Geometry check sheet. Reference: drawing and pictorial views, mm from the part's lowest x, y, z. Give positions to 0.01 mm unless a question says otherwise; leave off trailing zeros. Write each loop counter-clockwise with the first axis right and the second up, starting at its lowest first coordinate (ties: lowest second). Pieces come first, ordered by that corner, then holes. Notation, with made-up numbers: (20.5, -22) - (62.5, -22) arc R16 cw to (62.5, -5) - close; hole circle Ø8 at (41, 8.5). An arc over 180 degrees is marked (long way). Put each result on its own line as item: value.
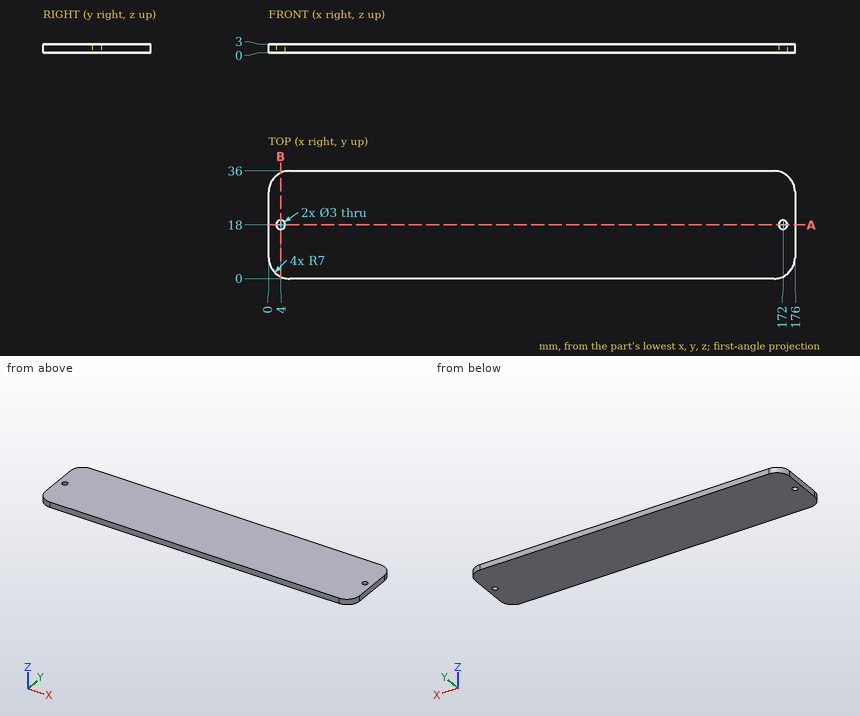
Q1. Go/stop test with a flat-tipped pin: pin 1 Ø1 at (y, z) = (5, 0.5) entering from +X. Record where the tip stops, or that it passes through.
Answers follow:
pin 1: stops at x = 175.84
Q2. Section check B-B, the plane x = 4. Record the cut outline in (y, z).
Answers follow:
outline: (0.68, 0) - (16.5, 0) - (16.5, 3) - (0.68, 3) - close; (19.5, 0) - (35.32, 0) - (35.32, 3) - (19.5, 3) - close
Q3. Scan lines: line 1 along Y through (x, z) = (4, 1.25); line 2 along X through (y, z) = (2, 2.6); line 3 along X through (y, z) = (33, 2.35). Record each from-to range of solid material in increasing order.
Answers follow:
line 1: y = 0.68 to 16.5, 19.5 to 35.32
line 2: x = 2.1 to 173.9
line 3: x = 1.26 to 174.74
Q4. Section check A-A, the plane y = 18. Record the cut outline in (x, z).
Answers follow:
outline: (0, 0) - (2.5, 0) - (2.5, 3) - (0, 3) - close; (5.5, 0) - (170.5, 0) - (170.5, 3) - (5.5, 3) - close; (173.5, 0) - (176, 0) - (176, 3) - (173.5, 3) - close
